```python
from build123d import *

# Parameters (mm, degrees)
F0_W     = 60
F0_H     = 54
F0_W_2   = 54
F0_H_2   = 48
F1_DEPTH = 3
F2_DEPTH = 3
F3_R     = 2.5
F4_DEPTH = 2
F5_R     = 1.5
F6_DEPTH = 3


with BuildPart() as f1:
    # F0 (on Top) → F1 (new body)
    with BuildSketch(Plane.XY):
        Rectangle(F0_W, F0_H)
        Rectangle(F0_W_2, F0_H_2, mode=Mode.SUBTRACT)
        Rectangle(F0_W_2, F0_H_2)
    extrude(amount=-F1_DEPTH)

    # F0 (on Top) → F2 (join)
    with BuildSketch(Plane.XY):
        Rectangle(F0_W, F0_H)
        Rectangle(F0_W_2, F0_H_2, mode=Mode.SUBTRACT)
    extrude(amount=F2_DEPTH)

    # F3 (on face) → F4 (cut)
    with BuildSketch(Plane.XY):
        with Locations((-18, 15)):
            Circle(F3_R)
        with Locations((18, 15)):
            Circle(F3_R)
        with Locations((18, -15)):
            Circle(F3_R)
        with Locations((-18, -15)):
            Circle(F3_R)
    extrude(amount=-F4_DEPTH, mode=Mode.SUBTRACT)

    # F5 (on face) → F6 (cut, through all)
    with BuildSketch(Plane.XY):
        with Locations((-23, 20)):
            Circle(F5_R)
        with Locations((23, 20)):
            Circle(F5_R)
        with Locations((-23, -20)):
            Circle(F5_R)
        with Locations((23, -20)):
            Circle(F5_R)
    extrude(amount=-F6_DEPTH, mode=Mode.SUBTRACT)


solid = f1.part
```
Design review of the part built by this model. Coordinates are the model's own, in mm. A direction names the side the tool comes from. Coordinates: 2 decimals unless noted, no trailing zeros. Loops run counter-clockwise (first coordinate to the right, second up) from the corner with the lowest first, then second, coordinate; pieces in that order, holes last. Notation, with made-up numbers: (15.25, 35.5) - (44.25, 35.5) arc R14 ccw to (44.25, 53.5) - close; hole circle Ø6 at (5, 88). An arc over 180 degrees is marked (long way). Use CSV: the item, a comma, the result in double quotes. Start each with the question number.
1) Consider section D-D on y = 20. Write out the cut boundary in (x, z).
2) Tool access review of faces 1 (the cylindrical face through (21.89, 21.01, -1.48)), 2 (the cylindrical face through (-20.5, -14.9, -1)): name each direction out of +Z, -Z, +X, -X, +Y, -Y from which nothing blocks a thin tool from reaching the whole face with its end or side.
3) Consider section A-A on y = -15. Write out the cut boundary in (x, z), then the cut area to 3 significant figures.
4) Consider section B-B on z = 1.5. Write out the cut boundary in (x, y).
5) For pin 1 Ø5.5 at (x, y) = (-17, -15.5) entering from +Z; pin 2 Ø1.8 at (x, y) = (23, -20) entering from -Z; pin 3 Ø2.5 at (x, y) = (-19, 14.5) entering from +Z, all flat-tipped, find the tip position at first contact; note any pin that passes through.
6) The part is to be moulded in two halves that separate along X. For faces 3 (the flat face through (0, -27, 0)), 4 (the flat face through (18, -15, -2)), 5 (the flat face through (30, 0, 0)), say which applies: +X half, -X half, draft (parallel to the pull), parting line (faces both ways), or undercut.
7) Wall thickness on L1, parallel to Y at x = 23, z = -1.8; L2, parallel to Y at x = 18, z = -0.4; L3, parallel to Y at x = 15, z = 2.7: over which ranges is each line inside the solid? List them lowest first. Write a range as from..to.
8) Consider section C-C on x = -23. Write out the cut boundary in (y, z), then the cut area to 3 significant figures.
Geometry says:
1,outline,"(-30, -3) - (-24.5, -3) - (-24.5, 0) - (-27, 0) - (-27, 3) - (-30, 3) - close; (-21.5, -3) - (21.5, -3) - (21.5, 0) - (-21.5, 0) - close; (24.5, -3) - (30, -3) - (30, 3) - (27, 3) - (27, 0) - (24.5, 0) - close"
2,face 1,"+Z, -Z"
2,face 2,"+Z"
3,outline,"(-30, -3) - (30, -3) - (30, 3) - (27, 3) - (27, 0) - (20.5, 0) - (20.5, -2) - (15.5, -2) - (15.5, 0) - (-15.5, 0) - (-15.5, -2) - (-20.5, -2) - (-20.5, 0) - (-27, 0) - (-27, 3) - (-30, 3) - close"
3,area,"178 mm^2"
4,outline,"(-30, -27) - (30, -27) - (30, 27) - (-30, 27) - close; hole (-27, -24) - (27, -24) - (27, 24) - (-27, 24) - close"
5,pin 1,"z = 0"
5,pin 2,"through"
5,pin 3,"z = -2"
6,face 3,"draft"
6,face 4,"undercut"
6,face 5,"+X half"
7,L1,"-27..-21.5, -18.5..18.5, 21.5..27"
7,L2,"-27..-17.5, -12.5..12.5, 17.5..27"
7,L3,"-27..-24, 24..27"
8,outline,"(-27, -3) - (-21.5, -3) - (-21.5, 0) - (-24, 0) - (-24, 3) - (-27, 3) - close; (-18.5, -3) - (18.5, -3) - (18.5, 0) - (-18.5, 0) - close; (21.5, -3) - (27, -3) - (27, 3) - (24, 3) - (24, 0) - (21.5, 0) - close"
8,area,"162 mm^2"
